The drawing under review shows one solid part. Ordinate dimensions are in mm from its lowest x, y, z. A direction names the side the tool comes from. Give positions to 0.01 mm unless a question says otherwise; leave off trailing zeros. Write each loop counter-clockwise with the first axis right and the second up, starting at its lowest first coordinate (ties: lowest second). Pieces come first, ordered by that corner, then holes. Notation, with made-up numbers: M 68,60.5 L 87,60.5 A31 ccw 87,97.5 Z; hole C 58,-26.5 d10. An arc over 180 degrees is marked long. Write item = value, one per line. Start each with the question number.
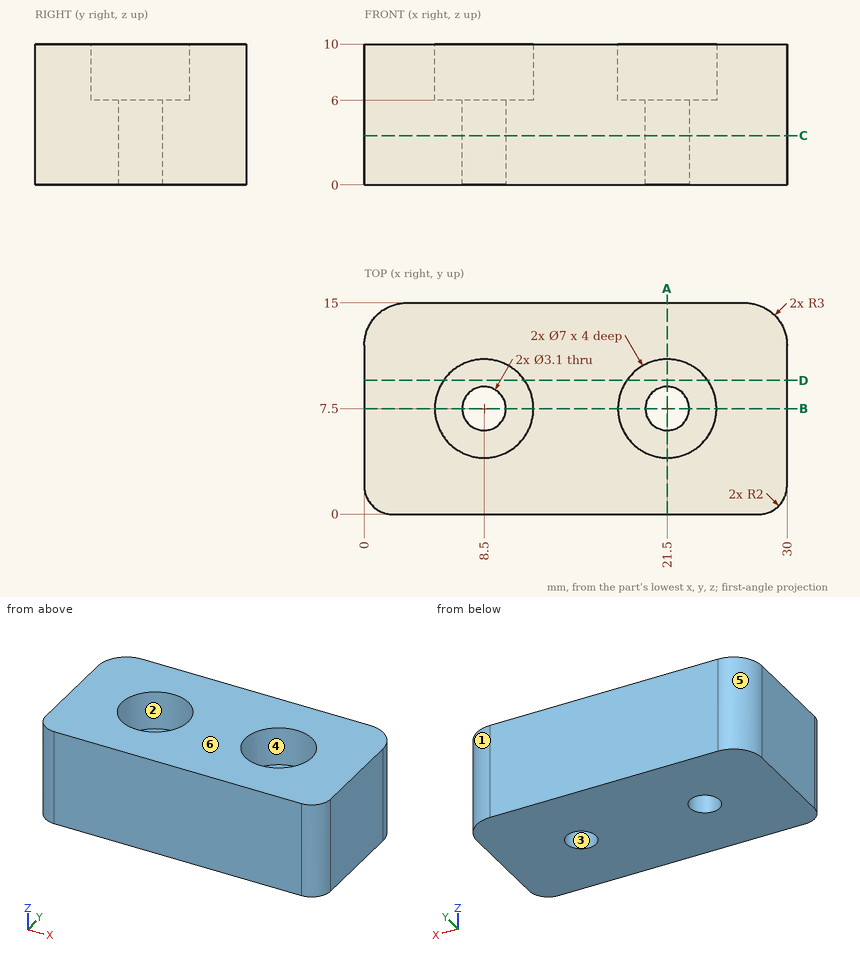
Item 1: We need section B-B, the plane y = 7.5. Write out the cut boundary in (x, z), and give its area (3 significant figures).
Item 2: Clearance check with flat-ended pins moving along their axes: P1, Ø3.5, axis at x = 20.5, y = 6, coming from the +Z side; P2, Ø3.5, axis at x = 8.5, y = 7.5, coming from the +Z side. State where each tip first meets the part, or that it passes through.
Item 3: We need section C-C, the plane z = 3.5. Write out the cut boundary in (x, y), and give its area (3 significant figures).
Item 4: We need section D-D, the plane y = 9.5. Write out the cut boundary in (x, z).
Item 5: For the marked faces 1 and 2, list the 3-axis set-ups (+Z, -Z, +X, -X, +Y, -Y) from which the entire face can be reached by the end or side of a thin tool; tool diameter is ignored.
Item 6: To check wall thickness, follow probe 1 along Y at (x, z) = (8.5, 8.1); probe 2 along Y at (x, z) = (21.5, 2.5); probe 3 along X at (y, z) = (7, 9.75). State the ranges of each line that lie inside material, in increasing order. Write a range as [from, to].
Item 7: We need section A-A, the plane x = 21.5. Write out the cut boundary in (y, z).
Item 8: The part is to be moulded in two halves that separate along X. For the marked faces 3, 4, 5 and 6, say which applies: released by +X, released by -X, zero draft, split by the parting line, or undercut.
Worked out:
q1.outline = M 0,0 L 6.95,0 L 6.95,6 L 5,6 L 5,10 L 0,10 Z; M 10.05,0 L 19.95,0 L 19.95,6 L 18,6 L 18,10 L 12,10 L 12,6 L 10.05,6 Z; M 23.05,0 L 30,0 L 30,10 L 25,10 L 25,6 L 23.05,6 Z
q1.area = 207 mm²
q2.P1 = 10
q2.P2 = 6
q3.outline = M 0,2 A2 ccw 2,0 L 28,0 A2 ccw 30,2 L 30,12 A3 ccw 27,15 L 3,15 A3 ccw 0,12 Z; hole C 8.5,7.5 d3.1; hole C 21.5,7.5 d3.1
q3.area = 429 mm²
q4.outline = M 0,0 L 30,0 L 30,10 L 24.37,10 L 24.37,6 L 18.63,6 L 18.63,10 L 11.37,10 L 11.37,6 L 5.63,6 L 5.63,10 L 0,10 Z
q5.face_1 = +Z, -Z, +X, +Y
q5.face_2 = +Z
q6.probe_1 = [0, 4], [11, 15]
q6.probe_2 = [0, 5.95], [9.05, 15]
q6.probe_3 = [0, 5.04], [11.96, 18.04], [24.96, 30]
q7.outline = M 0,0 L 5.95,0 L 5.95,6 L 4,6 L 4,10 L 0,10 Z; M 9.05,0 L 15,0 L 15,10 L 11,10 L 11,6 L 9.05,6 Z
q8.face_3 = undercut
q8.face_4 = undercut
q8.face_5 = released by -X
q8.face_6 = zero draft
